CAD build for the part. Positions are in the model's coordinates, mm. A direction names the side the tool comes from. Give positions to 0.01 mm unless a question says otherwise; leave off trailing zeros. Write each loop counter-clockwise with the first axis right and the second up, starting at its lowest first coordinate (ties: lowest second). Pieces come first, ordered by that corner, then holes. Notation, with made-up numbers: (79.5, 32) - (97.5, 32) arc R26 cw to (97.5, 59) - close; hole circle Ø5 at (58, -17.75). An arc over 180 degrees is marked (long way). Put each result on its own line as item: value. Start each with the question number.
1. Cut at A-A on z = 0. List the corners of the cut face in (x, y).
2. Cut at B-B on x = 0. List the corners of the cut face in (y, z).
3. Drop flat-ended pins along their axis: pin 1 (2 mm diameter, centred on y = 63, z = -13.5, fed in from +X); pin 2 (5 mm diameter, centred on y = 36, z = -22, fed in from +X); pin 3 (6 mm diameter, centred on x = -4, y = -16, fed in from +Z). Give the stop position or say it passes through.
4. Mould opens along Z. For faces 5 (the conical face through (7.16, 40.56, -32.243)), 6 (the cylindrical face through (-30.05, 2.01, 0.18)), 7 (the flat face through (10, -19, 12)) say: +Z half, -Z half, draft (parallel to the pull), parting line (faces both ways), or undercut.
5. Tool access for faces 1 (the flat face through (-0.1, 0, 31.3)), 2 (the flat face through (1, 2, 0)), 3 (the flat face through (0, -19, 32)), 4 (the cylindrical face through (-3.534, -19.375, 0.156)): list every direction of +Z, -Z, +X, -X, +Y, -Y with a clear straight run to the whole face (end or side of a thin tool).
6. Cut at C-C on y = -5. List the corners of the cut face in (x, z), and give its area (3 significant figures).
7. Wall check: line 1 (Z direction, x = 0, y = -13); line 2 (Y direction, x = -6, z = -20); line 3 (Z direction, x = 6, y = 11). Give the ranges that are in metal, low to high.
from build123d import *

# Parameters (mm, degrees)
SKETCH2_R           = 12.5
CUT_EXTRUDE1_DEPTH  = 10
SKETCH3_W           = 20
SKETCH3_H           = 40
SKETCH3_R           = 3.537482137
BOSS_EXTRUDE1_DEPTH = 39.3


with BuildPart() as part:
    # Sketch1 → Revolve1 (revolve)
    with BuildSketch(Plane.XY):
        Polygon((0, 0), (-31, 0), (-35, 80), (-33.002495322, 80.099875234), (-29.097501561, 2), (0, 2), align=None)
    revolve(axis=Axis((0, 0, 0), (0, 1, 0)))

    # Sketch2 → Cut-Extrude1 (cut)
    with BuildSketch(Plane.XZ):
        with Locations((-17.550020437, 0)):
            Circle(SKETCH2_R)
    extrude(amount=-CUT_EXTRUDE1_DEPTH, mode=Mode.SUBTRACT)

    # Sketch3 → Boss-Extrude1 (add)
    with BuildSketch(Plane.XZ):
        with Locations((0, 12)):
            Rectangle(SKETCH3_W, SKETCH3_H)
        Circle(SKETCH3_R, mode=Mode.SUBTRACT)
    extrude(amount=BOSS_EXTRUDE1_DEPTH)


solid = part.part
Report:
1. outline: (-35, 80) - (-31, 0) - (-30.05, 0) - (-30.05, 10) - (-29.5, 10) - (-33, 80.1) - close; (-10, -39.3) - (-3.54, -39.3) - (-3.54, 0) - (3.54, 0) - (3.54, -39.3) - (10, -39.3) - (10, 0) - (31, 0) - (35, 80) - (33, 80.1) - (29.1, 2) - (-5.05, 2) - (-5.05, 0) - (-10, 0) - close
2. outline: (-39.3, -8) - (0, -8) - (0, -31) - (80, -35) - (80.1, -33) - (2, -29.1) - (2, 29.1) - (80.1, 33) - (80, 35) - (0, 31) - (0, 32) - (-39.3, 32) - (-39.3, 3.54) - (0, 3.54) - (0, -3.54) - (-39.3, -3.54) - close
3. pin 1: stops at x = 31.78
3. pin 2: stops at x = 26.38
3. pin 3: stops at z = 32
4. face 5: parting line
4. face 6: undercut
4. face 7: draft
5. face 1: +Z
5. face 2: +Y
5. face 3: +Z, +X, -X, -Y
5. face 4: -Y
6. outline: (-10, -8) - (10, -8) - (10, 32) - (-10, 32) - close; hole circle Ø7.07 at (0, 0)
6. area: 761 mm²
7. line 1: z = -8 to -3.54, 3.54 to 32
7. line 2: y = 0 to 2
7. line 3: z = -30.97 to -28.93, 28.93 to 30.97
